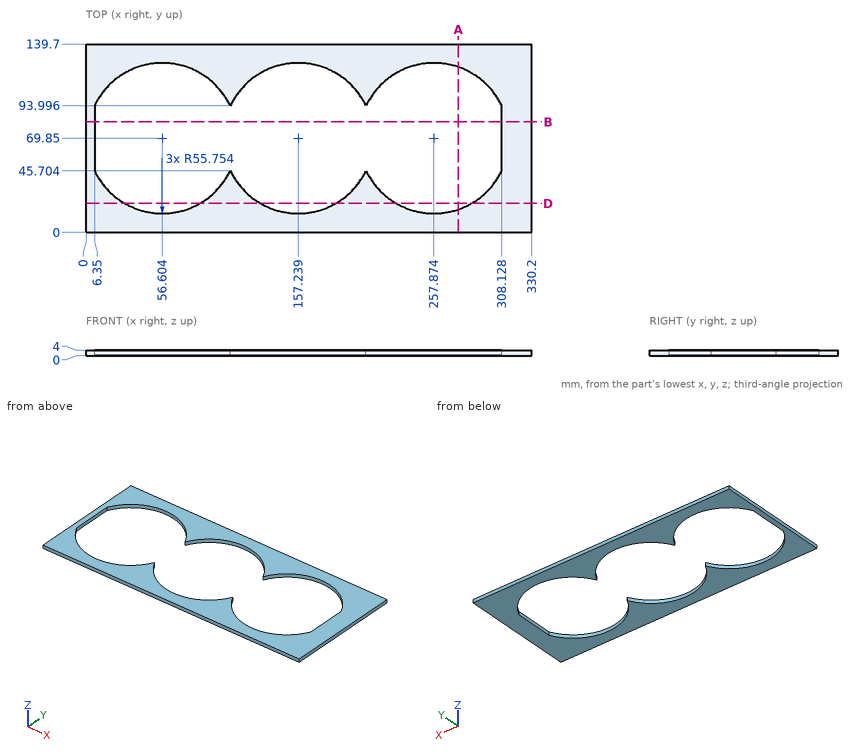
Here's the drawing with two shaded views (mm, measured from the low corner). I have some questions. Give positions to 0.01 mm unless a question says otherwise; leave off trailing zeros. Loops run counter-clockwise (first coordinate to the right, second up) from the corner with the lowest first, then second, coordinate; pieces in that order, holes last. Notation, with made-up numbers: (2.5, 5.5) -> (17.5, 5.5) arc R13 cw to (17.5, 15.5) -> close; hole circle Ø2 at (58, 28). An arc over 180 degrees is marked (long way). Answer as a JSON object with one key per item and string values. Group by question number.
Item 1: I need wall thicknesses on L1, parallel to X at y = 59.5, z = 0.8; L2, parallel to Y at x = 156, z = 1.1; L3, parallel to X at y = 27, z = 0.4 (1 decimal). Which ranges of each line are inside material? Lowest first, please.
Item 2: Imagine slicing it at D-D on y = 21.5. Write out the boundary of the cut face in (x, z).
Item 3: Imagine slicing it at A-A on x = 276. Write out the boundary of the cut face in (y, z) (1 decimal), then the cut area to 3 significant figures.
Item 4: Imagine slicing it at B-B on y = 82. Write out the boundary of the cut face in (x, z), then the cut area to 3 significant figures.
Item 5: Will this pin go through, and if not, where does the flat tip stop? pin 1 (1 mm diameter, centred on y = 54.5, z = 1, fed in from -X).
Answer list:
{
 "1": {"L1": "x = 0 to 6.35, 308.13 to 330.2", "L2": "y = 0 to 14.11, 125.59 to 139.7", "L3": "x = 0 to 20.9, 92.3 to 121.6, 192.9 to 222.2, 293.5 to 330.2"},
 "2": {"outline": "(0, 0) -> (28.84, 0) -> (28.84, 4) -> (0, 4) -> close; (84.37, 0) -> (129.48, 0) -> (129.48, 4) -> (84.37, 4) -> close; (185, 0) -> (230.11, 0) -> (230.11, 4) -> (185, 4) -> close; (285.64, 0) -> (330.2, 0) -> (330.2, 4) -> (285.64, 4) -> close"},
 "3": {"outline": "(0, 0) -> (17.1, 0) -> (17.1, 4) -> (0, 4) -> close; (122.6, 0) -> (139.7, 0) -> (139.7, 4) -> (122.6, 4) -> close", "area": "137 mm2"},
 "4": {"outline": "(0, 0) -> (6.35, 0) -> (6.35, 4) -> (0, 4) -> close; (308.13, 0) -> (330.2, 0) -> (330.2, 4) -> (308.13, 4) -> close", "area": "114 mm2"},
 "5": {"pin 1": "stops at x = 0"}
}
